For this review, use the dimensioned drawing (mm, ordinates from the lowest corner) and the shaded views. A direction names the side the tool comes from. Give positions to 0.01 mm unless a question says otherwise; leave off trailing zeros. Loops run counter-clockwise (first coordinate to the right, second up) from the corner with the lowest first, then second, coordinate; pieces in that order, holes last. Notation, with made-up numbers: (37.5, -6.75) - (83.5, -6.75) arc R28 cw to (83.5, 15.25) - close; hole circle Ø9 at (-9.5, -21). An arc over 180 degrees is marked (long way). Write each question's results on one line, items separated by ' | '.
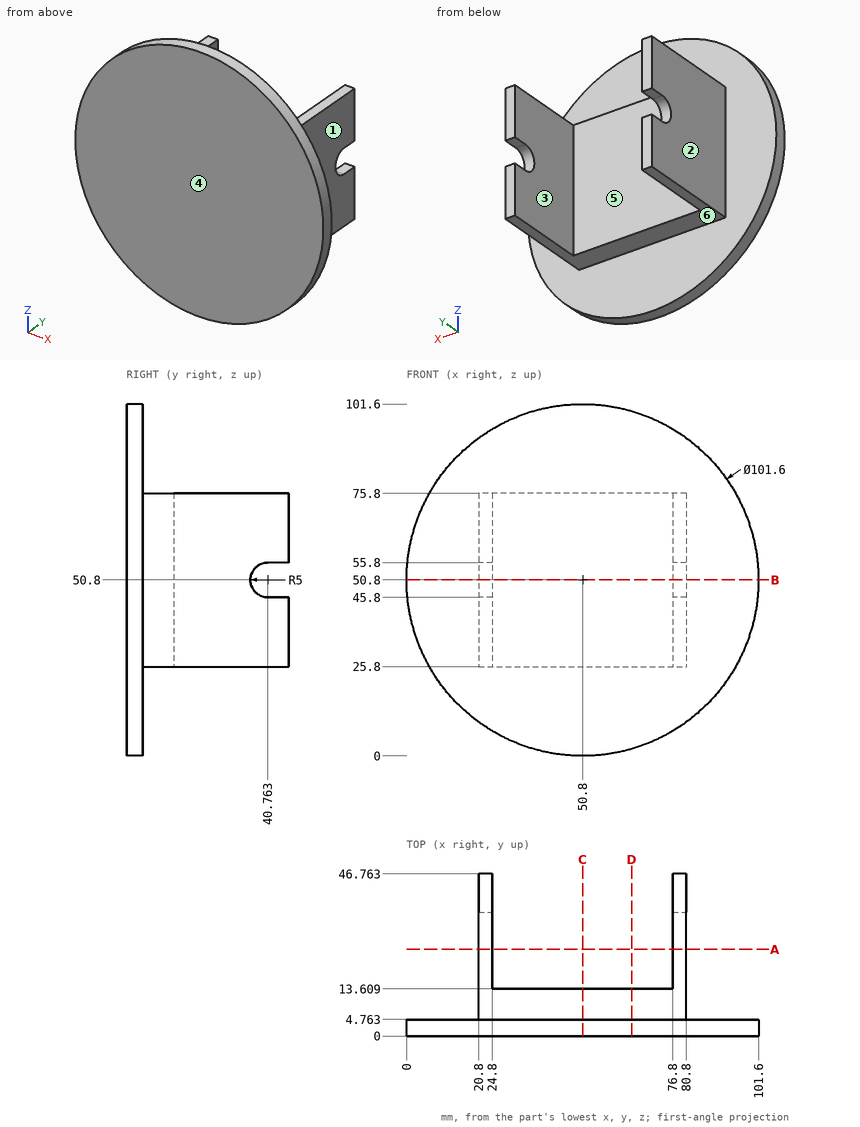
Item 1: Wall thickness on probe 1 along X at (y, z) = (21.5, 50.5); probe 2 along Z at (x, y) = (32.5, 12); probe 3 along Y at (x, z) = (36, 82.5): over which ranges is each line inside the solid? List them lowest first.
Output values:
probe 1: x = 20.8 to 24.8, 76.8 to 80.8 | probe 2: z = 25.8 to 75.8 | probe 3: y = 0 to 4.76
Item 2: We need section C-C on x = 50.8. Give the boundary of the cut face in (y, z), then the cut area to 3 significant figures.
Output values:
outline: (0, 0) - (4.76, 0) - (4.76, 25.8) - (13.61, 25.8) - (13.61, 75.8) - (4.76, 75.8) - (4.76, 101.6) - (0, 101.6) - close | area: 926 mm²
Item 3: We need section A-A on y = 25. Give the boundary of the cut face in (x, z), then the cut area to 3 significant figures.
Output values:
outline: (20.8, 25.8) - (24.8, 25.8) - (24.8, 75.8) - (20.8, 75.8) - close; (76.8, 25.8) - (80.8, 25.8) - (80.8, 75.8) - (76.8, 75.8) - close | area: 400 mm²
Item 4: Tool access review of the marked faces 4, 5 and 6: name each direction out of +Z, -Z, +X, -X, +Y, -Y from which nothing blocks a thin tool from reaching the whole face with its end or side.
Output values:
face 4: +Z, -Z, +X, -X, -Y | face 5: +Z, -Z, +Y | face 6: -Z, +X, -X, +Y
Item 5: Draft analysis for pull direction X (two halves, no side actions). For the marked faces 1, 2 and 3, state which applies: +X half, -X half, draft (parallel to the pull), parting line (faces both ways), or undercut.
Output values:
face 1: +X half | face 2: -X half | face 3: undercut
Item 6: Clearance check with flat-ended pins moving along their axes: P1, Ø3, axis at x = 31, z = 66.5, coming from the +Y side; P2, Ø10, axis at y = 12, z = 31, coming from the +X side; P3, Ø3, axis at x = 38, z = 84.5, coming from the +Y side. State where each tip first meets the part, or that it passes through.
Output values:
P1: stops at y = 13.61 | P2: stops at x = 80.8 | P3: stops at y = 4.76
Item 7: We need section B-B on z = 50.8. Give the boundary of the cut face in (x, y).
Output values:
outline: (0, 0) - (101.6, 0) - (101.6, 4.76) - (80.8, 4.76) - (80.8, 35.76) - (76.8, 35.76) - (76.8, 13.61) - (24.8, 13.61) - (24.8, 35.76) - (20.8, 35.76) - (20.8, 4.76) - (0, 4.76) - close
Item 8: We need section D-D on x = 65. Give the boundary of the cut face in (y, z) (1 decimal).
Output values:
outline: (0, 2) - (4.8, 2) - (4.8, 25.8) - (13.6, 25.8) - (13.6, 75.8) - (4.8, 75.8) - (4.8, 99.6) - (0, 99.6) - close
